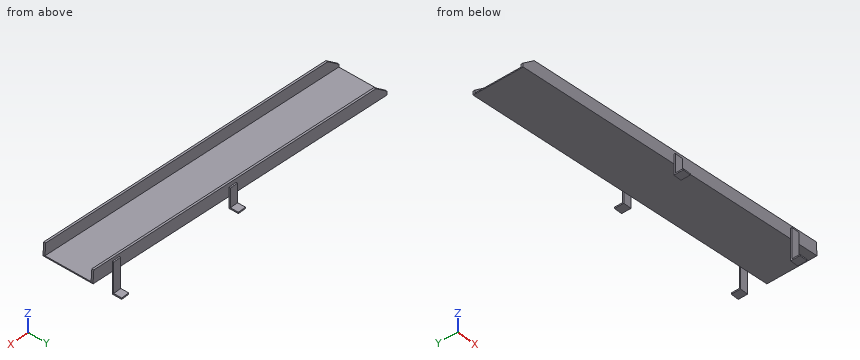
```python
from build123d import *

# Parameters (mm, degrees)
F1_DEPTH = 187.5
F2_W     = 2506.2565537025
F2_H     = 15
F3_DEPTH = 90
F4_W     = 60
F4_H     = 10
F5_DEPTH = 70
F4_H_2   = 228.9615774155
F4_H_3   = 143.8855462986
F6_DEPTH = 10
F9_DEPTH = 375


with BuildPart() as f1:
    # F0 (on Front) → F1 (new body, symmetric)
    with BuildSketch(Plane.XZ):
        Polygon((-1084.3461751938, 8.0200209718), (-1084.3461751938, 0), (1415.6538248062, 176.9799790282), (1415.6538248062, 185), align=None)
    extrude(amount=F1_DEPTH, both=True)

    # F2 (on face) → F3 (join)
    with BuildSketch(Plane(origin=(-5.9720318293, 0, 84.3602742827), x_dir=(0.997503626, 0, 0.0706152683), z_dir=(-0.0706152683, 0, 0.997503626))):
        with Locations((172.0553711911, -180)):
            Rectangle(F2_W, F2_H)
        with Locations((172.0553711911, 180)):
            Rectangle(F2_W, F2_H)
    extrude(amount=F3_DEPTH)



with BuildPart() as f5:
    # F4 (on face) → F5 (new body)
    with BuildSketch(Plane.XZ.offset(187.5)):
        with Locations((228.0231494724, 13.0200209718)):
            Rectangle(F4_W, F4_H)
    extrude(amount=F5_DEPTH)


with BuildPart() as f5b:
    # F4 (on face) → F5, piece 2 (new body)
    with BuildSketch(Plane.XZ.offset(187.5)):
        with Locations((1221.529750824, 5)):
            Rectangle(F4_W, F4_H)
    extrude(amount=F5_DEPTH)


with BuildPart() as f1_1:
    add(f1.part)

    add(f5.part)  # F6 merges F5

    add(f5b.part)  # F6 merges F5b
    # F4 (on face) → F6 (join)
    with BuildSketch(Plane.XZ.offset(187.5)):
        with Locations((1221.529750824, 124.4807887077)):
            Rectangle(F4_W, F4_H_2)
        with Locations((1221.529750824, 5)):
            Rectangle(F4_W, F4_H)
        with Locations((228.0231494724, 89.9627941211)):
            Rectangle(F4_W, F4_H_3)
        with Locations((228.0231494724, 13.0200209718)):
            Rectangle(F4_W, F4_H)
    extrude(amount=F6_DEPTH)

    # F7: F1 across plane


with BuildPart() as f1_2:
    add(f1_1.part)
    add(f1_1.part.mirror(Plane.XZ))

    # F8 (on face) → F9 (cut, through all)
    with BuildSketch(Plane.XZ.offset(187.5)):
        Polygon((-1085.7584805603, 27.9700934918), (-990.9511867431, 104.8568741441), (-1090.7015493429, 97.7953473117), align=None)
    extrude(amount=-F9_DEPTH, mode=Mode.SUBTRACT)


solid = f1_2.part
```
Can you work these out from the model? Positions are in its coordinate system, mm. Coordinates: 2 decimals unless noted, no trailing zeros. Write each loop counter-clockwise with the first axis right and the second up, starting at its lowest first coordinate (ties: lowest second). Pieces come first, ordered by that corner, then holes. Notation, with made-up numbers: M -7,47.5 L 41,47.5 A33 ccw 41,78.5 Z; hole C 35.5,-7.75 d3. An arc over 180 degrees is marked long. Write item = value, one per line. Start each with the question number.
Q1. If I drill on L1, parallel to Y at x = 1258.5, z = 263; L2, parallel to Z at x = -667.5, y = 86; L3, parallel to Z at x = 591.5, y = -134.5, over which ranges is the centre line in solid material (lowest first)? Write a range as [from, to].
Q2. If we section it at C-C, the plane x = -484: Write out the boundary of the cut face in (y, z), then the cut area to 3 significant figures.
Q3. If we section it at D-D, the plane y = 2.5: Write out the boundary of the cut face in (x, z).
Q4. If we section it at B-B, the plane z = 214: Write out the boundary of the cut face in (x, y), then the cut area to 3 significant figures.
Q5. If we section it at A-A, the plane y = -225: Write out the boundary of the cut face in (x, z), then the cut area to 3 significant figures.
Q6. I'm going to push flat-ended pins straight in: pin 1 (18 mm diameter, centred on x = 1228.5, z = 132.5, fed in from -Y); pin 2 (6 mm diameter, centred on x = -544.5, z = 87, fed in from +Y); pin 3 (18 mm diameter, centred on x = 242.5, z = 88, fed in from +Y). Where does each tip first touch, or does it pass through?
Check sheet entries:
q1.L1 = [-187.5, -172.5], [172.5, 187.5]
q1.L2 = [29.51, 37.53]
q1.L3 = [118.64, 126.66]
q2.outline = M -187.5,42.5 L 187.5,42.5 L 187.5,140.74 L 172.5,140.74 L 172.5,50.52 L -172.5,50.52 L -172.5,140.74 L -187.5,140.74 Z
q2.area = 5,710 mm²
q3.outline = M -1084.35,0 L 1415.65,176.98 L 1415.65,185 L -1084.35,8.02 Z
q4.outline = M 550.79,-187.5 L 1191.53,-187.5 L 1191.53,-197.5 L 1251.53,-197.5 L 1251.53,-187.5 L 1413.6,-187.5 L 1413.6,-172.5 L 550.79,-172.5 Z; M 550.79,172.5 L 1413.6,172.5 L 1413.6,187.5 L 1251.53,187.5 L 1251.53,197.5 L 1191.53,197.5 L 1191.53,187.5 L 550.79,187.5 Z
q4.area = 27,100 mm²
q5.outline = M 198.02,8.02 L 258.02,8.02 L 258.02,18.02 L 198.02,18.02 Z; M 1191.53,0 L 1251.53,0 L 1251.53,10 L 1191.53,10 Z
q5.area = 1,200 mm²
q6.pin_1 = -197.5
q6.pin_2 = 187.5
q6.pin_3 = 197.5
